Design review of the part shown in the three views and the two pictorial views. Dimensions are in mm from the part's minimum x, y and z. Coordinates: 2 decimals unless noted, no trailing zeros. Loops run counter-clockwise (first coordinate to the right, second up) from the corner with the lowest first, then second, coordinate; pieces in that order, holes last. Notation, with made-up numbers: (55.25, -1) -> (114.25, -1) arc R10 ccw to (114.25, 5) -> close; hole circle Ø3 at (68.25, 14.25). An arc over 180 degrees is marked (long way). One line per item, written item: value.
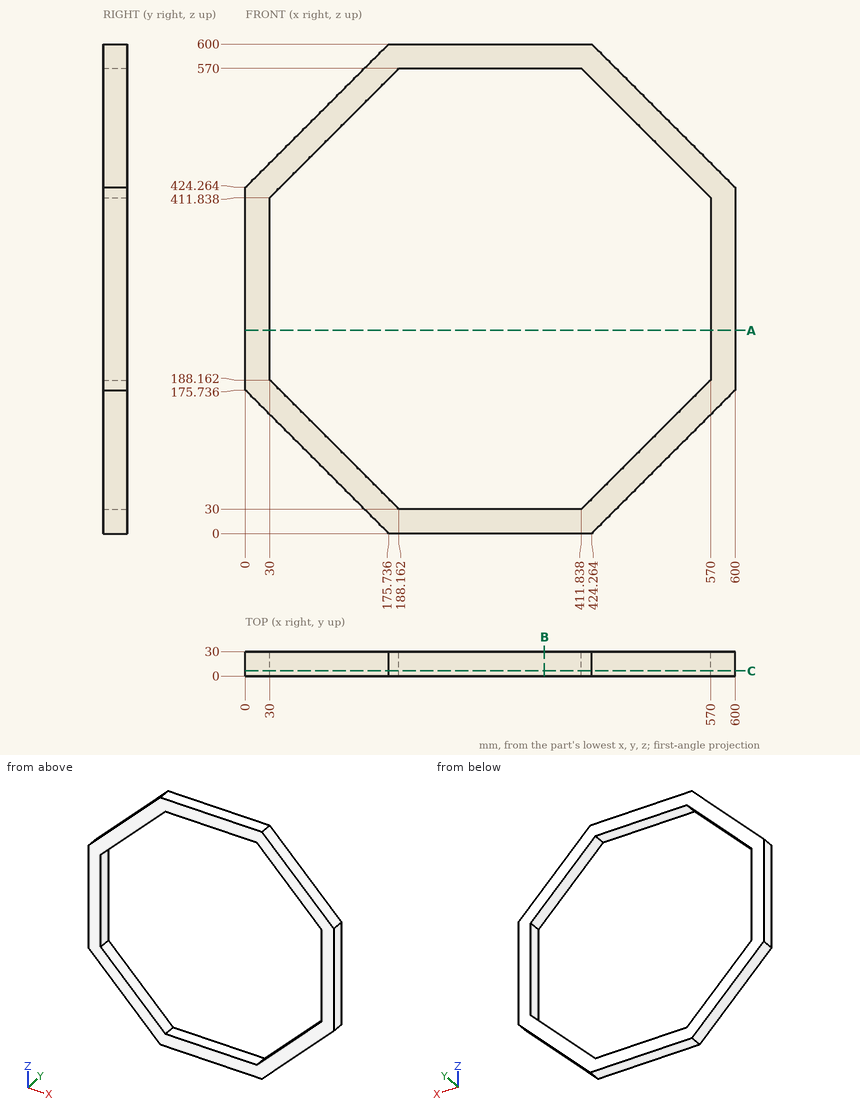
1. To check wall thickness, follow probe 1 along Z at (x, y) = (404.5, 21.5); probe 2 along X at (y, z) = (22.5, 88.5) (1 decimal). State the ranges of each line that lie inside material, in increasing order. Write a range as from..to.
Return value:
probe 1: z = 0..30, 570..600
probe 2: x = 87.2..129.7, 470.3..512.8
2. Take a section at C-C, the plane y = 6.25. Give the boundary of the cut face in (x, z), and give its area (3 significant figures).
Return value:
outline: (0, 175.74) -> (175.74, 0) -> (424.26, 0) -> (600, 175.74) -> (600, 424.26) -> (424.26, 600) -> (175.74, 600) -> (0, 424.26) -> close; hole (30, 188.16) -> (188.16, 30) -> (411.84, 30) -> (570, 188.16) -> (570, 411.84) -> (411.84, 570) -> (188.16, 570) -> (30, 411.84) -> close
area: 56,700 mm2
3. Take a section at A-A, the plane z = 249. Give the boundary of the cut face in (x, y).
Return value:
outline: (0, 0) -> (30, 0) -> (30, 30) -> (0, 30) -> close; (570, 0) -> (600, 0) -> (600, 30) -> (570, 30) -> close
4. Take a section at B-B, the plane x = 366.5. Give the boundary of the cut face in (y, z), and give its area (3 significant figures).
Return value:
outline: (0, 0) -> (30, 0) -> (30, 30) -> (0, 30) -> close; (0, 570) -> (30, 570) -> (30, 600) -> (0, 600) -> close
area: 1,800 mm2
5. Insertion check: pin 1 Ø10 at (x, z) = (80, 513) entering from +Y; pin 2 Ø10 at (x, y) = (146, 16.5) entering from +Z (1 decimal). Each pin has a flat end and moves straight along its axis. Give the tip position at first contact, or say it passes through.
Return value:
pin 1: passes through
pin 2: stops at z = 575.3
